Input: part model. Units: mm. Frame: model coordinates. Coordinates: 2 decimals unless noted, no trailing zeros. Order: outer loops, then holes, each group sorted by start corner. A loop starts at its lowest first (then second) coordinate and runs counter-clockwise, first axis right, second up.
from build123d import *

# Parameters (mm, degrees)
F0_W           = 89.2
F0_H           = 36
F1_DEPTH       = 5
F2_D           = 6.6
F2_DEPTH       = 15
F2_TIP         = 1.9828400428
F3_D           = 3.4
F3_DEPTH       = 15
F3_CSINK_D     = 6.5
F3_CSINK_ANGLE = 90
F3_TIP         = 1.0214630523
F4_R           = 2
F5_SIZE        = 0.5


with BuildPart() as f1:
    # F0 (on Top) → F1 (new body)
    with BuildSketch(Plane.XY):
        Rectangle(F0_W, F0_H)
    extrude(amount=F1_DEPTH)

    # F2
    with Locations(Plane(origin=(0, 0, 0), x_dir=(1, 0, 0), z_dir=(0, 0, -1))):
        with Locations((-35.4, 0), (-10.4, 0), (14.6, 0), (29.6, 0)):
            Hole(F2_D / 2, depth=F2_DEPTH)
            with Locations((0, 0, -(F2_DEPTH + F2_TIP / 2))):  # 118° drill point
                Cone(0, F2_D / 2, F2_TIP, mode=Mode.SUBTRACT)

    # F3
    with Locations(Plane(origin=(0, 0, 0), x_dir=(1, 0, 0), z_dir=(0, 0, -1))):
        with Locations((-40.6, 13), (-40.6, -13), (39.6, -13), (39.6, 13)):
            CounterSinkHole(F3_D / 2, F3_CSINK_D / 2, depth=F3_DEPTH, counter_sink_angle=F3_CSINK_ANGLE)
            with Locations((0, 0, -(F3_DEPTH + F3_TIP / 2))):  # 118° drill point
                Cone(0, F3_D / 2, F3_TIP, mode=Mode.SUBTRACT)

    # F4
    f4_edges = [f1.edges().sort_by_distance(p)[0] for p in [
        (-44.6, 18, 2.5),
        (44.6, 18, 2.5),
        (-44.6, -18, 2.5),
        (44.6, -18, 2.5),
    ]]
    fillet(f4_edges, radius=F4_R)

    # F5
    f5_edges = [f1.edges().sort_by_distance(p)[0] for p in [
        (44.6, 0, 0),
    ]]
    chamfer(f5_edges, length=F5_SIZE)


solid = f1.part
Item 1: Cut plane C-C on x = 29.6. Return loops of the section in (y, z).
Response values:
outline: (-18, 0.5) - (-17.5, 0) - (-3.3, 0) - (-3.3, 5) - (-18, 5) - close; (3.3, 0) - (17.5, 0) - (18, 0.5) - (18, 5) - (3.3, 5) - close
Item 2: Draft query along X for faces 1 (the face through (-44.6, 0, 3)), 2 (the face through (-38.9, 12.93, 3.3)), 3 (the face through (-1, -18, 3)). Return one class per face: pulls with the +X half, pulls with the -X half, needs draft (parallel to the pull), parting line crosses it, or undercut.
Response values:
face 1: pulls with the -X half
face 2: undercut
face 3: needs draft
Item 3: Ray query, probe 1 along X at (y, z) = (-13, 2.7); probe 2 along Y at (x, z) = (39.6, 4.15); probe 3 along Y at (x, z) = (14.6, 1.95). Return the intervals inside material, ascending.
Response values:
probe 1: x = -44.6 to -42.3, -38.9 to 37.9, 41.3 to 44.6
probe 2: y = -18 to -14.7, -11.3 to 11.3, 14.7 to 18
probe 3: y = -18 to -3.3, 3.3 to 18
Item 4: Pin query (flat end, axial travel): pin 1 Ø5.5 at (x, y) = (39.6, -13) entering from -Z; pin 2 Ø10 at (x, y) = (-16.5, 14.5) entering from -Z. Return the tip coordinate at first contact, or that it passes through.
Response values:
pin 1: stops at z = 0.5
pin 2: stops at z = 0
Item 5: Cut plane A-A on y = 13. Return loops of the section in (x, z), then the cut area to 3 significant figures.
Response values:
outline: (-44.6, 0.5) - (-44.1, 0) - (-43.85, 0) - (-42.3, 1.55) - (-42.3, 5) - (-44.6, 5) - close; (-38.9, 1.55) - (-37.35, 0) - (36.35, 0) - (37.9, 1.55) - (37.9, 5) - (-38.9, 5) - close; (41.3, 1.55) - (42.85, 0) - (44.1, 0) - (44.6, 0.5) - (44.6, 5) - (41.3, 5) - close
area: 407 mm2
Item 6: Cut plane D-D on y = 0. Return loops of the section in (x, z), then the cut area to 3 significant figures.
Response values:
outline: (-44.6, 0.5) - (-44.1, 0) - (-38.7, 0) - (-38.7, 5) - (-44.6, 5) - close; (-32.1, 0) - (-13.7, 0) - (-13.7, 5) - (-32.1, 5) - close; (-7.1, 0) - (11.3, 0) - (11.3, 5) - (-7.1, 5) - close; (17.9, 0) - (26.3, 0) - (26.3, 5) - (17.9, 5) - close; (32.9, 0) - (44.1, 0) - (44.6, 0.5) - (44.6, 5) - (32.9, 5) - close
area: 314 mm2
Item 7: Cut plane B-B on z = 3.75. Count the separate pieces of the cut face and the enclosed holes in it, then the cut area to 3 significant figures.
Response values:
separate pieces: 1
enclosed holes: 8
area: 3,030 mm2
